Design review of the part built by this model. Coordinates are the model's own, in mm. A direction names the side the tool comes from. Coordinates: 2 decimals unless noted, no trailing zeros. Loops run counter-clockwise (first coordinate to the right, second up) from the corner with the lowest first, then second, coordinate; pieces in that order, holes last. Notation, with made-up numbers: M -11.75,82 L 24.25,82 A21 cw 24.25,118 Z; hole C -12.5,-13 d6. An arc over 180 degrees is marked long. Answer as a JSON object with one key per item and string values. Group by question number.
1. Draft analysis for pull direction Z (two halves, no side actions). For faces 5 (the flat face through (0, 2, 55)), 6 (the flat face through (-18, -18, 9.75)), 7 (the flat face through (5, -2, 42.35)), state which applies: +Z half, -Z half, draft (parallel to the pull), parting line (faces both ways), or undercut.
2. Consider section B-B (y = -12). State the section outline as (x, z) points, then the cut area to 3 significant figures.
3. Insertion check: pin 1 (3 mm diameter, centred on x = -15, y = -15.5, fed in from +Z); pin 2 (1.2 mm diameter, centred on x = 15.5, y = -15, fed in from +Z); pin 3 (12 mm diameter, centred on x = -12, z = 45.5, fed in from +Y). Each pin has a flat end and moves straight along its axis. Give the tip position at first contact, or say it passes through.
4. Machinability: for faces 1 (the flat face through (18, -18, 9.75)), 2 (the flat face through (18, 18, 32.75)), 3 (the cylindrical face through (14.579, 16.345, 38.401)), 4 (the flat face through (-18, 18, 32.75)), which of the approach directions +Z, -Z, +X, -X, +Y, -Y give a long, thin tool a straight path to every point of the face, cutting with its end or side? Answer none if there is none.
5. Consider section A-A (z = 13). State the section outline as (x, y) points.
6. To check wall thickness, follow probe 1 along Y at (x, z) = (-15.5, 39.15); probe 2 along Y at (x, z) = (0, 41.3) (3 decimals); probe 3 along Z at (x, y) = (-4.5, -6). State the ranges of each line that lie inside material, in increasing order.
7. Consider section C-C (z = 49). State the section outline as (x, y) points.
from build123d import *

# Parameters (mm, degrees)
SKETCH_1_W          = 42
SKETCH_1_H          = 42
EXTRUDE_1_DEPTH     = 40.5
SKETCH_2_W          = 16
SKETCH_2_H          = 4
EXTRUDE_2_DEPTH     = 3.15
CUT_EXTRUDE_1_REACH = 54.022
CUT_EXTRUDE_START   = -9.75
CUT_EXTRUDE_2_DEPTH = 23
SKETCH_5_R          = 11
SKETCH_5_R_2        = 4.875
EXTRUDE_4_DEPTH     = 1.85
SKETCH_6_R          = 4.75
SKETCH_6_R_2        = 2.625
EXTRUDE_5_DEPTH     = 0.5
CHAMFER_1_SIZE      = 0.2
SKETCH_7_R          = 2.5
EXTRUDE_6_DEPTH     = 23.5
SKETCH_8_R          = 1.25
CUT_EXTRUDE_3_DEPTH = 4
CHAMFER_2_SIZE      = 0.25
CUT_EXTRUDE_START_2 = -18
CUT_EXTRUDE_4_DEPTH = 18
CHAMFER_3_SIZE      = 0.5
FILLET_1_R          = 0.25
FILLET_2_R          = 1.5
FILLET_3_R          = 2
FILLET_4_R          = 0.5


with BuildPart() as part:
    # 草图1 → 凸台-拉伸1 (new body)
    with BuildSketch(Plane.XY):
        Rectangle(SKETCH_1_W, SKETCH_1_H)
    extrude(amount=EXTRUDE_1_DEPTH)

    # 草图2 → 凸台-拉伸2 (add)
    with BuildSketch(Plane(origin=(0, 0, 0), x_dir=(-1, 0, 0), z_dir=(0, 0, -1))):
        with Locations((0, 23)):
            Rectangle(SKETCH_2_W, SKETCH_2_H)
    extrude(amount=-EXTRUDE_2_DEPTH)

    # 草图3 → 切除-拉伸1 (cut, up to next)
    with BuildSketch(Plane(origin=(0, 0, 0), x_dir=(-1, 0, 0), z_dir=(0, 0, -1)), mode=Mode.PRIVATE) as cut_extrude_1_sk1:
        Polygon((-17.075, 21), (-21, 17.075), (-21, 21), align=None)
    cut_extrude_1_tool1 = extrude(cut_extrude_1_sk1.sketch, amount=-CUT_EXTRUDE_1_REACH, mode=Mode.PRIVATE) & part.part
    # 草图3 → 切除-拉伸1 (cut, up to next)
    with BuildSketch(Plane(origin=(0, 0, 0), x_dir=(-1, 0, 0), z_dir=(0, 0, -1)), mode=Mode.PRIVATE) as cut_extrude_1_sk2:
        Polygon((17.075, 21), (21, 17.075), (21, 21), align=None)
    cut_extrude_1_tool2 = extrude(cut_extrude_1_sk2.sketch, amount=-CUT_EXTRUDE_1_REACH, mode=Mode.PRIVATE) & part.part
    # 草图3 → 切除-拉伸1 (cut, up to next)
    with BuildSketch(Plane(origin=(0, 0, 0), x_dir=(-1, 0, 0), z_dir=(0, 0, -1)), mode=Mode.PRIVATE) as cut_extrude_1_sk3:
        Polygon((21, -17.075), (17.075, -21), (21, -21), align=None)
    cut_extrude_1_tool3 = extrude(cut_extrude_1_sk3.sketch, amount=-CUT_EXTRUDE_1_REACH, mode=Mode.PRIVATE) & part.part
    # 草图3 → 切除-拉伸1 (cut, up to next)
    with BuildSketch(Plane(origin=(0, 0, 0), x_dir=(-1, 0, 0), z_dir=(0, 0, -1)), mode=Mode.PRIVATE) as cut_extrude_1_sk4:
        Polygon((-21, -17.075), (-17.075, -21), (-21, -21), align=None)
    cut_extrude_1_tool4 = extrude(cut_extrude_1_sk4.sketch, amount=-CUT_EXTRUDE_1_REACH, mode=Mode.PRIVATE) & part.part
    add(cut_extrude_1_tool1.solids().sort_by_distance((19.691667, 19.691667, 0))[0], mode=Mode.SUBTRACT)
    add(cut_extrude_1_tool2.solids().sort_by_distance((-19.691667, 19.691667, 0))[0], mode=Mode.SUBTRACT)
    add(cut_extrude_1_tool3.solids().sort_by_distance((-19.691667, -19.691667, 0))[0], mode=Mode.SUBTRACT)
    add(cut_extrude_1_tool4.solids().sort_by_distance((19.691667, -19.691667, 0))[0], mode=Mode.SUBTRACT)

    # 草图4 → 切除-拉伸2 (cut)
    with BuildSketch(Plane(origin=(0, 0, 0), x_dir=(-1, 0, 0), z_dir=(0, 0, -1)).offset(CUT_EXTRUDE_START)):
        Polygon((-21, 14.532), (-14.532, 21), (-21, 21), align=None)
        Polygon((14.532, 21), (21, 14.532), (21, 21), align=None)
        Polygon((21, -14.532), (14.532, -21), (21, -21), align=None)
        Polygon((-14.532, -21), (-21, -14.532), (-21, -21), align=None)
    extrude(amount=-CUT_EXTRUDE_2_DEPTH, mode=Mode.SUBTRACT)

    # 草图5 → 凸台-拉伸4 (add)
    with BuildSketch(Plane.XY.offset(40.5)):
        Circle(SKETCH_5_R)
        Circle(SKETCH_5_R_2, mode=Mode.SUBTRACT)
    extrude(amount=EXTRUDE_4_DEPTH)

    # 草图6 → 凸台-拉伸5 (add)
    with BuildSketch(Plane.XY.offset(40.5)):
        Circle(SKETCH_6_R)
        Circle(SKETCH_6_R_2, mode=Mode.SUBTRACT)
    extrude(amount=EXTRUDE_5_DEPTH)

    # 倒角1
    chamfer_1_edges = [part.edges().sort_by_distance(p)[0] for p in [
        (-4.75, 0, 41),
        (-2.625, 0, 41),
    ]]
    chamfer(chamfer_1_edges, length=CHAMFER_1_SIZE)

    # 草图7 → 凸台-拉伸6 (add)
    with BuildSketch(Plane.XY.offset(40.5)):
        Circle(SKETCH_7_R)
    extrude(amount=EXTRUDE_6_DEPTH)

    # 草图8 → 切除-拉伸3 (cut)
    with BuildSketch(Plane.XY.offset(40.5)):
        with Locations((-15.5, 15.5)):
            Circle(SKETCH_8_R)
        with Locations((15.5, 15.5)):
            Circle(SKETCH_8_R)
        with Locations((15.5, -15.5)):
            Circle(SKETCH_8_R)
        with Locations((-15.5, -15.5)):
            Circle(SKETCH_8_R)
    extrude(amount=-CUT_EXTRUDE_3_DEPTH, mode=Mode.SUBTRACT)

    # 倒角2
    chamfer_2_edges = [part.edges().sort_by_distance(p)[0] for p in [
        (-16.75, -15.5, 40.5),
        (14.25, -15.5, 40.5),
        (14.25, 15.5, 40.5),
        (-16.75, 15.5, 40.5),
    ]]
    chamfer(chamfer_2_edges, length=CHAMFER_2_SIZE)

    # 草图9 → 切除-拉伸4 (cut)
    with BuildSketch(Plane.XY.offset(64).offset(CUT_EXTRUDE_START_2)):
        with BuildLine():
            Line((-1.5, 2), (1.5, 2))
            ThreePointArc((1.5, 2), (0, 2.5), (-1.5, 2))
        make_face()
    extrude(amount=CUT_EXTRUDE_4_DEPTH, mode=Mode.SUBTRACT)

    # 倒角3
    chamfer_3_edges = [part.edges().sort_by_distance(p)[0] for p in [
        (-1.118033989, -2.236067977, 64),
    ]]
    chamfer(chamfer_3_edges, length=CHAMFER_3_SIZE - 0.0001)  # a hair under: the kernel refuses the full size

    # 圆角1
    fillet_1_edges = [part.edges().sort_by_distance(p)[0] for p in [
        (-11, 0, 42.35),
    ]]
    fillet(fillet_1_edges, radius=FILLET_1_R)

    # 圆角2
    fillet_2_edges = [part.edges().sort_by_distance(p)[0] for p in [
        (21, -17.075, 36.625),
        (17.075, -21, 36.625),
        (-21, -17.075, 36.625),
        (-17.075, -21, 36.625),
        (-17.075, 21, 36.625),
        (-21, 17.075, 36.625),
        (17.075, 21, 36.625),
        (21, 17.075, 36.625),
        (17.075, -21, 4.875),
        (21, -17.075, 4.875),
        (-21, -17.075, 4.875),
        (-17.075, -21, 4.875),
        (-17.075, 21, 4.875),
        (-21, 17.075, 4.875),
        (21, 17.075, 4.875),
        (17.075, 21, 4.875),
    ]]
    fillet(fillet_2_edges, radius=FILLET_2_R)

    # 圆角3
    fillet_3_edges = [part.edges().sort_by_distance(p)[0] for p in [
        (-21, -14.532, 21.25),
        (-14.532, -21, 21.25),
        (-14.532, 21, 21.25),
        (-21, 14.532, 21.25),
        (21, 14.532, 21.25),
        (14.532, 21, 21.25),
        (14.532, -21, 21.25),
        (21, -14.532, 21.25),
    ]]
    fillet(fillet_3_edges, radius=FILLET_3_R)

    # 圆角4
    fillet_4_edges = [part.edges().sort_by_distance(p)[0] for p in [
        (-12.226839828, 21, 0),
        (-8, 23, 0),
        (0, 25, 0),
        (8, 23, 0),
        (-21, 0, 0),
        (0, -21, 0),
        (21, 0, 0),
        (19.0375, -19.0375, 0),
        (-19.0375, -19.0375, 0),
        (-19.0375, 19.0375, 0),
        (12.226839828, 21, 0),
        (19.0375, 19.0375, 0),
        (17.027704805, 20.885819299, 0),
        (20.885819299, 17.027704805, 0),
        (20.885819299, -17.027704805, 0),
        (17.027704805, -20.885819299, 0),
        (-20.885819299, 17.027704805, 0),
        (-17.027704805, 20.885819299, 0),
        (-20.885819299, -17.027704805, 0),
        (-17.027704805, -20.885819299, 0),
    ]]
    fillet(fillet_4_edges, radius=FILLET_4_R)


solid = part.part
Findings below:
{
 "1": {"face 5": "draft", "face 6": "undercut", "face 7": "+Z half"},
 "2": {"outline": "M -21,0.5 A0.5 ccw -20.5,0 L 20.5,0 A0.5 ccw 21,0.5 L 21,40.5 L -21,40.5 Z", "area": "1,700 mm^2"},
 "3": {"pin 1": "stops at z = 40.5", "pin 2": "stops at z = 36.5", "pin 3": "stops at y = 21"},
 "4": {"face 1": "+X, -Y", "face 2": "+X, +Y", "face 3": "+Z", "face 4": "-X, +Y"},
 "5": {"outline": "M -21,-13.7 A2 ccw -20.41,-15.12 L -15.12,-20.41 A2 ccw -13.7,-21 L 13.7,-21 A2 ccw 15.12,-20.41 L 20.41,-15.12 A2 ccw 21,-13.7 L 21,13.7 A2 ccw 20.41,15.12 L 15.12,20.41 A2 ccw 13.7,21 L -13.7,21 A2 ccw -15.12,20.41 L -20.41,15.12 A2 ccw -21,13.7 Z"},
 "6": {"probe 1": "y = -21 to -16.75, -14.25 to 14.25, 16.75 to 21", "probe 2": "y = -11 to -4.875, -2.5 to 2.5, 4.875 to 11", "probe 3": "z = 0 to 42.35"},
 "7": {"outline": "M -1.5,2 A2.5 ccw long 1.5,2 Z"}
}
